Geometry: final body of the model. Coordinates: model frame, mm. Face numbers are marked on the shaded views. A direction names the side the tool comes from. Round coordinates to 2 decimals unless told otherwise and drop trailing zeros. Loops run counter-clockwise (first coordinate to the right, second up) from the corner with the lowest first, then second, coordinate; pieces in that order, holes last. Notation, with made-up numbers: M 28.25,4 L 75.25,4 A29 cw 75.25,27 Z; hole C 25.25,45 d8. An arc over 180 degrees is marked long. Write each question's results on one line, items separated by ' | '.
```python
from build123d import *

# Parameters (mm, degrees)
SKETCH_1_R               = 3.5
EXTRUDE_1_DEPTH          = 20
SKETCH_2_R               = 1.5
CUT_EXTRUDE_1_DEPTH      = 10
SKETCH_3_R               = 1
CUT_EXTRUDE_2_DEPTH      = 10
SKETCH_4_R               = 4.5
SKETCH_4_R_2             = 3.5
EXTRUDE_2_DEPTH          = 6
EXTRUDE_START            = -6
SKETCH_5_R               = 4.5
SKETCH_5_R_2             = 3.5
EXTRUDE_3_DEPTH          = 6
CHAMFER_1_SIZE           = 0.58
CHAMFER_1_SIZE_2         = 1.004589468
CUT_EXTRUDE_3_DEPTH      = 21.988091862
CUT_EXTRUDE_3_DEPTH_BACK = 21.988091862
SKETCH_6_R               = 1.5


with BuildPart() as part:
    # 草圖1 → 填料-伸長1 (new body)
    with BuildSketch(Plane(origin=(0, 0, 0), x_dir=(1, 0, 0), z_dir=(0, 1, 0))):
        with Locations(Location((0, 0, 0), (0, 0, 270))):
            Circle(SKETCH_1_R)
    extrude(amount=EXTRUDE_1_DEPTH)

    # 草圖2 → 除料-伸長1 (cut)
    with BuildSketch(Plane(origin=(0, 20, 0), x_dir=(1, 0, 0), z_dir=(0, 1, 0))):
        with Locations(Location((0, 0, 0), (0, 0, 270))):
            Circle(SKETCH_2_R)
    extrude(amount=-CUT_EXTRUDE_1_DEPTH, mode=Mode.SUBTRACT)

    # 草圖3 → 除料-伸長2 (cut)
    with BuildSketch(Plane.XZ):
        with Locations(Location((0, 0, 0), (0, 0, 270))):
            Circle(SKETCH_3_R)
    extrude(amount=-CUT_EXTRUDE_2_DEPTH, mode=Mode.SUBTRACT)

    # 草圖4 → 填料-伸長2 (add)
    with BuildSketch(Plane.XZ):
        with Locations(Location((0, 0, 0), (0, 0, 270))):
            Circle(SKETCH_4_R)
        with Locations(Location((0, 0, 0), (0, 0, 270))):
            Circle(SKETCH_4_R_2, mode=Mode.SUBTRACT)
    extrude(amount=-EXTRUDE_2_DEPTH)

    # 草圖5 → 填料-伸長3 (add)
    with BuildSketch(Plane(origin=(0, 20, 0), x_dir=(1, 0, 0), z_dir=(0, 1, 0)).offset(EXTRUDE_START)):
        with Locations(Location((0, 0, 0), (0, 0, 90))):
            Circle(SKETCH_5_R)
        with Locations(Location((0, 0, 0), (0, 0, 90))):
            Circle(SKETCH_5_R_2, mode=Mode.SUBTRACT)
    extrude(amount=EXTRUDE_3_DEPTH)

    # 導角1
    # the kernel refuses this chamfer: 1.004589468, 0.58 mm, written as the material it adds along each edge
    with BuildSketch(Plane(origin=(0, 14, 0), x_dir=(0, 0, 1), z_dir=(1, 0, 0))) as chamfer_1_piece_1_section:
        Polygon((3.5, CHAMFER_1_SIZE), (3.5 + CHAMFER_1_SIZE_2, 0), (3.5, 0), align=None)
    chamfer_1_piece_1 = revolve(axis=Axis((0, 14, 0), (0, -1, 0)), mode=Mode.PRIVATE)
    chamfer_1_piece_1 = chamfer_1_piece_1 & Plane(origin=(0, 13.715905857, 0), x_dir=(0, 0, -1), z_dir=(0, -1, 0)) * Cylinder(4.5, 19, mode=Mode.PRIVATE)
    add(chamfer_1_piece_1)
    with BuildSketch(Plane(origin=(0, 6, 0), x_dir=(0, 0, 1), z_dir=(-1, 0, 0))) as chamfer_1_piece_2_section:
        Polygon((3.5, CHAMFER_1_SIZE), (3.5 + CHAMFER_1_SIZE_2, 0), (3.5, 0), align=None)
    chamfer_1_piece_2 = revolve(axis=Axis((0, 6, 0), (0, 1, 0)), mode=Mode.PRIVATE)
    chamfer_1_piece_2 = chamfer_1_piece_2 & Plane(origin=(0, 6.284094143, 0), x_dir=(0, 0, -1), z_dir=(0, -1, 0)) * Cylinder(4.5, 19, mode=Mode.PRIVATE)
    add(chamfer_1_piece_2)

    # 草圖6 → 除料-伸長3 (cut, two sides: drawn at the far end of the back side and taken through both)
    with BuildSketch(Plane.XY.offset(-CUT_EXTRUDE_3_DEPTH_BACK)):
        with Locations((0, 17)):
            Circle(SKETCH_6_R)
        with Locations((0, 3)):
            Circle(SKETCH_6_R)
    extrude(amount=CUT_EXTRUDE_3_DEPTH + CUT_EXTRUDE_3_DEPTH_BACK, mode=Mode.SUBTRACT)


solid = part.part
```
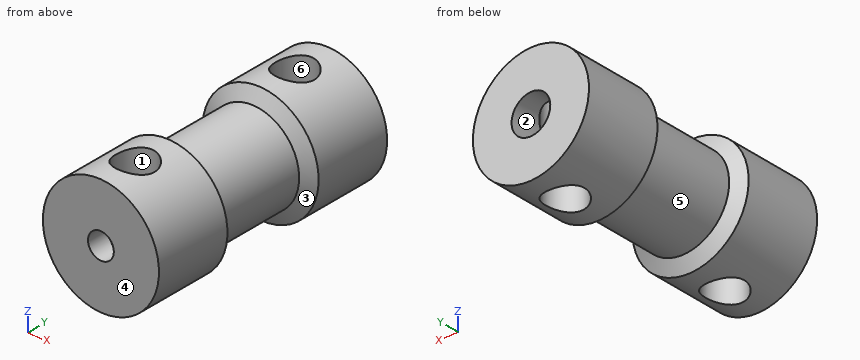
1. Access query for the marked faces 1, 2 and 3. Directions: +Z, -Z, +X, -X, +Y, -Y. A direction counts if a zero-diameter tool reaches every point of the face in a straight line with its end or side. Return the directions, or none.
Answer key:
face 1: +Z, -Z | face 2: +Y | face 3: none
2. Section B-B (x = 0). Count the separate pieces of the cut face and the enclosed holes in it, then the cut area to 3 significant figures.
Answer key:
separate pieces: 6 | enclosed holes: 0 | area: 76.2 mm²
3. Pin query (flat end, axial travel): P1, Ø1, axis at x = 1, y = 15.5, coming from the -Z side; P2, Ø5, axis at y = 8.5, z = 2.5, coming from the -X side; P3, Ø1.5, axis at x = -2.5, y = 12.5, coming from the +Z side. Return the tip coordinate at first contact, or that it passes through.
Answer key:
P1: stops at z = -4.47 | P2: stops at x = -3.94 | P3: stops at z = 3.03
4. Ray query, probe 1 along Z at (x, y) = (0, 12.5); probe 2 along Z at (x, y) = (0, 7.2). Return the intervals inside material, ascending.
Answer key:
probe 1: z = -3.5 to -1.5, 1.5 to 3.5 | probe 2: z = -3.5 to -1, 1 to 3.5
5. Section A-A (y = 11). Output: boundary loops of the cut face in (x, z).
Answer key:
outline: C 0,0 d7; hole C 0,0 d3
6. Section C-C (y = 3). Output: boundary loops of the cut face in (x, z), then the cut area to 3 significant figures.
Answer key:
outline: M -1.5,-4.24 L -1.5,4.24 A4.5 ccw Z; M 1.5,-4.24 A4.5 ccw 1.5,4.24 Z | area: 37.1 mm²
7. Draft query along X for the marked faces 4, 5 and 6. Return one class per face: pulls with the +X half, pulls with the -X half, needs draft (parallel to the pull), parting line crosses it, or undercut.
Answer key:
face 4: needs draft | face 5: parting line crosses it | face 6: undercut
